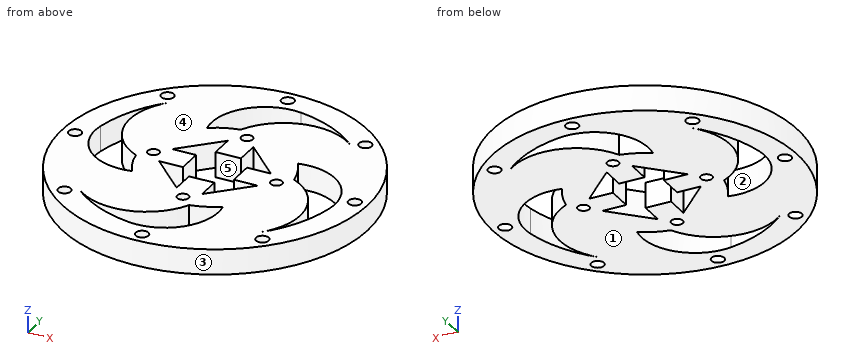
from build123d import *

# Parameters (mm, degrees)
SKETCH6_R                        = 29
SKETCH6_R_2                      = 20
INNER_RING_DEPTH                 = 10
MOTOR_CONNECTOR_CUT_DEPTH        = 10
SKETCH8_R                        = 2.25
MOTOR_CONNECTOR_HOLES_DEPTH      = 1
MOTOR_CONNECTOR_HOLES_DEPTH_BACK = 18
MIDDLE_PATTERN_DEPTH             = 10
SKETCH9_R                        = 60
SKETCH9_R_2                      = 50
SKETCH9_R_3                      = 2.5
BOSS_EXTRUDE1_DEPTH              = 10
BOSS_EXTRUDE2_DEPTH              = 10


with BuildPart() as part:
    # Sketch6 → Inner Ring (new body)
    with BuildSketch(Plane.XY):
        Circle(SKETCH6_R)
        Circle(SKETCH6_R_2, mode=Mode.SUBTRACT)
    extrude(amount=-INNER_RING_DEPTH)

    # Sketch7 → Motor Connector Cut (add)
    with BuildSketch(Plane.XY):
        with BuildLine():
            ThreePointArc((20, 0), (19.840593925, 2.52008585), (19.364916731, 5))
            Line((19.364916731, 5), (9.999996731, 5))
            Line((9.999996731, 5), (9.999996731, -5))
            Line((9.999996731, -5), (19.364916731, -5))
            ThreePointArc((19.364916731, -5), (19.840593925, -2.52008585), (20, 0))
        make_face()
        with BuildLine():
            ThreePointArc((5, 19.364916731), (0, 20), (-5, 19.364916731))
            Line((-5, 19.364916731), (-5, 9.999996731))
            Line((-5, 9.999996731), (5, 9.999996731))
            Line((5, 9.999996731), (5, 19.364916731))
        make_face()
        with BuildLine():
            Line((-9.999996731, -5), (-9.999996731, 5))
            Line((-9.999996731, 5), (-19.364916731, 5))
            ThreePointArc((-19.364916731, 5), (-20, 0), (-19.364916731, -5))
            Line((-19.364916731, -5), (-9.999996731, -5))
        make_face()
        with BuildLine():
            Line((-5, -9.999996731), (-5, -19.364916731))
            ThreePointArc((-5, -19.364916731), (0, -20), (5, -19.364916731))
            Line((5, -19.364916731), (5, -9.999996731))
            Line((5, -9.999996731), (-5, -9.999996731))
        make_face()
    extrude(amount=-MOTOR_CONNECTOR_CUT_DEPTH)

    # Sketch8 → Motor Connector Holes (cut, two sides)
    with BuildSketch(Plane.XY) as motor_connector_holes_sk:
        with Locations((0, 24.182458366)):
            Circle(SKETCH8_R)
        with Locations((24.182458366, 0)):
            Circle(SKETCH8_R)
        with Locations((0, -24.182458366)):
            Circle(SKETCH8_R)
        with Locations((-24.182458366, 0)):
            Circle(SKETCH8_R)
    extrude(amount=MOTOR_CONNECTOR_HOLES_DEPTH, mode=Mode.SUBTRACT)
    extrude(motor_connector_holes_sk.sketch, amount=-MOTOR_CONNECTOR_HOLES_DEPTH_BACK, mode=Mode.SUBTRACT)

    # Sketch10 → Middle Pattern (add)
    with BuildSketch(Plane.XY):
        with BuildLine():
            ThreePointArc((28.607215414, 4.756808408), (26.539406056, -11.690163651), (15.800414568, -24.317625284))
            ThreePointArc((15.800414568, -24.317625284), (10.393277118, -43.149392299), (-8.201394307, -49.322785114))
            ThreePointArc((-8.201394307, -49.322785114), (15.267827816, -47.611904328), (35.355339059, -35.355339059))
            ThreePointArc((35.355339059, -35.355339059), (42.321804958, -13.559663633), (28.607215414, 4.756808408))
        make_face()
        with BuildLine():
            ThreePointArc((24.317625284, 15.800414568), (43.149392359, 10.39327706), (49.322785087, -8.201394473))
            ThreePointArc((49.322785087, -8.201394473), (47.611904354, 15.267827736), (35.355339059, 35.355339059))
            ThreePointArc((35.355339059, 35.355339059), (13.559663633, 42.321804958), (-4.756808408, 28.607215414))
            ThreePointArc((-4.756808408, 28.607215414), (11.690163651, 26.539406056), (24.317625284, 15.800414568))
        make_face()
        with BuildLine():
            ThreePointArc((8.201394106, 49.322785148), (-15.267827902, 47.611904301), (-35.355339044, 35.355339075))
            ThreePointArc((-35.355339044, 35.355339075), (-42.32180496, 13.559663644), (-28.607215414, -4.756808408))
            ThreePointArc((-28.607215414, -4.756808408), (-26.539406056, 11.690163651), (-15.800414568, 24.317625284))
            ThreePointArc((-15.800414568, 24.317625284), (-10.393277189, 43.149392225), (8.201394106, 49.322785148))
        make_face()
        with BuildLine():
            ThreePointArc((4.756808408, -28.607215414), (-11.690163651, -26.539406056), (-24.317625284, -15.800414568))
            ThreePointArc((-24.317625284, -15.800414568), (-43.149392012, -10.393277393), (-49.322785244, 8.201393524))
            ThreePointArc((-49.322785244, 8.201393524), (-47.61190416, -15.267828343), (-35.355338839, -35.35533928))
            ThreePointArc((-35.355338839, -35.35533928), (-13.559663479, -42.321804932), (4.756808408, -28.607215414))
        make_face()
    extrude(amount=-MIDDLE_PATTERN_DEPTH)

    # Sketch9 → Boss-Extrude1 (add)
    with BuildSketch(Plane.XY):
        Circle(SKETCH9_R)
        Circle(SKETCH9_R_2, mode=Mode.SUBTRACT)
        with Locations((0, 55)):
            Circle(SKETCH9_R_3, mode=Mode.SUBTRACT)
        with Locations((-38.890872965, 38.890872965)):
            Circle(SKETCH9_R_3, mode=Mode.SUBTRACT)
        with Locations((-55, 0)):
            Circle(SKETCH9_R_3, mode=Mode.SUBTRACT)
        with Locations((-38.890872965, -38.890872965)):
            Circle(SKETCH9_R_3, mode=Mode.SUBTRACT)
        with Locations((0, -55)):
            Circle(SKETCH9_R_3, mode=Mode.SUBTRACT)
        with Locations((38.890872965, -38.890872965)):
            Circle(SKETCH9_R_3, mode=Mode.SUBTRACT)
        with Locations((55, 0)):
            Circle(SKETCH9_R_3, mode=Mode.SUBTRACT)
        with Locations((38.890872965, 38.890872965)):
            Circle(SKETCH9_R_3, mode=Mode.SUBTRACT)
    extrude(amount=-BOSS_EXTRUDE1_DEPTH)

    # Sketch11 → Boss-Extrude2 (add)
    with BuildSketch(Plane.XY):
        with BuildLine():
            Line((-19.364916731, 5), (-5, 19.364916731))
            ThreePointArc((-5, 19.364916731), (-14.142135624, 14.142135624), (-19.364916731, 5))
        make_face()
        with BuildLine():
            Line((5, 19.364916731), (19.364916731, 5))
            ThreePointArc((19.364916731, 5), (14.142135624, 14.142135624), (5, 19.364916731))
        make_face()
        with BuildLine():
            Line((19.364916731, -5), (5, -19.364916731))
            ThreePointArc((5, -19.364916731), (14.142135624, -14.142135624), (19.364916731, -5))
        make_face()
        with BuildLine():
            Line((-5, -19.364916731), (-19.364916731, -5))
            ThreePointArc((-19.364916731, -5), (-14.142135624, -14.142135624), (-5, -19.364916731))
        make_face()
    extrude(amount=-BOSS_EXTRUDE2_DEPTH)


solid = part.part
Here's how the part is built. I have some questions about the finished solid (model axes, mm). Face numbers are marked on the shaded views. A direction names the side the tool comes from. Coordinates: 2 decimals unless noted, no trailing zeros. Order: outer loops, then holes, each group sorted by start corner. A loop starts at its lowest first (then second) coordinate and runs counter-clockwise, first axis right, second up.
Item 1: For P1, Ø6, axis at x = 9.5, z = -6, coming from the +Y side; P2, Ø3, axis at y = -13, z = -5, coming from the -X side; P3, Ø4.5, axis at x = -38.89, y = -38.89, coming from the +Z side; P4, Ø5, axis at x = 2.5, z = -6.5, coming from the +Y side, each with a flat end and sliding along its axis, tell me the tip position at first contact or that it passes through.
Result sheet:
P1: stops at y = 59.65
P2: stops at x = -58.89
P3: passes through
P4: stops at y = 60
Item 2: If we section it at A-A on y = 0: State how many separate pieces and enclosed holes the cut face has, plus the area to 3 significant figures.
Result sheet:
separate pieces: 8
enclosed holes: 0
area: 535 mm2
Item 3: For the marked faces 4 and 5, which set-ups out of +Z, -Z, +X, -X, +Y, -Y let a thin tool reach every point of the face, with its end or its side?
Result sheet:
face 4: +Z, +X, -X, +Y, -Y
face 5: +Z, -Z
Item 4: I need wall thicknesses on line 1 (X direction, y = 31, z = -2.5); line 2 (X direction, y = -39.5, z = -2); line 3 (Y direction, x = 18, z = -1.75). Which ranges of each line are inside material? Lowest first, please.
Result sheet:
line 1: x = -51.37 to -39.23, -38.83 to -16.11, -3.43 to 51.37
line 2: x = -45.16 to -41.32, -36.47 to -30.66, -29.87 to -5.53, 13.2 to 36.47, 41.32 to 45.16
line 3: y = -57.24 to -6.36, -5 to 5, 6.36 to 42.67, 46.65 to 57.24
Item 5: If we mould it in two halves opening along Y, with no side actions, what happens to the marked faces 1, 2 and 3? For each: +Y half, -Y half, draft (parallel to the pull), parting line (faces both ways), or undercut.
Result sheet:
face 1: draft
face 2: undercut
face 3: parting line
Item 6: If we section it at B-B on y = 55: List the corners of the cut face in (x, z) for me, plus the area to 3 significant figures.
Result sheet:
outline: (-23.98, -10) - (-2.5, -10) - (-2.5, 0) - (-23.98, 0) - close; (2.5, -10) - (23.98, -10) - (23.98, 0) - (2.5, 0) - close
area: 430 mm2
